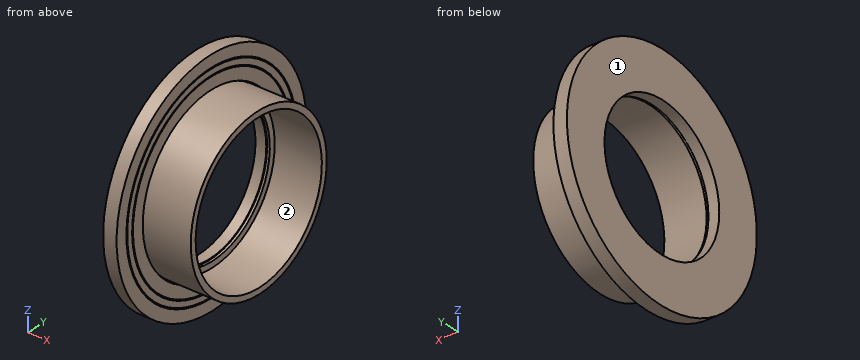
```python
from build123d import *

# Parameters (mm, degrees)
SKETCH1_R           = 17.08
SKETCH1_R_2         = 10.32
BOSS_EXTRUDE1_DEPTH = 2
SKETCH2_R           = 12.23
SKETCH2_R_2         = 11.35
BOSS_EXTRUDE2_DEPTH = 7
SKETCH3_R           = 10.47
SKETCH3_R_2         = 10.32
CUT_EXTRUDE1_DEPTH  = 0.4
SKETCH12_R          = 12.38
SKETCH12_R_2        = 12.23
CUT_EXTRUDE7_DEPTH  = 0.4
SKETCH13_R          = 14.29
SKETCH13_R_2        = 14.14
CUT_EXTRUDE8_DEPTH  = 0.4
SKETCH14_R          = 15.32
SKETCH14_R_2        = 15.17
CUT_EXTRUDE9_DEPTH  = 0.4


with BuildPart() as part:
    # Sketch1 → Boss-Extrude1 (new body)
    with BuildSketch(Plane(origin=(0, 0, 0), x_dir=(0, 0, -1), z_dir=(1, 0, 0))):
        Circle(SKETCH1_R)
        Circle(SKETCH1_R_2, mode=Mode.SUBTRACT)
    extrude(amount=BOSS_EXTRUDE1_DEPTH)

    # Sketch2 → Boss-Extrude2 (add)
    with BuildSketch(Plane(origin=(2, 0, 0), x_dir=(0, 0, -1), z_dir=(1, 0, 0))):
        Circle(SKETCH2_R)
        Circle(SKETCH2_R_2, mode=Mode.SUBTRACT)
    extrude(amount=BOSS_EXTRUDE2_DEPTH)

    # Sketch3 → Cut-Extrude1 (cut)
    with BuildSketch(Plane(origin=(2, 0, 0), x_dir=(0, 0, -1), z_dir=(1, 0, 0))):
        Circle(SKETCH3_R)
        Circle(SKETCH3_R_2, mode=Mode.SUBTRACT)
    extrude(amount=-CUT_EXTRUDE1_DEPTH, mode=Mode.SUBTRACT)

    # Sketch12 → Cut-Extrude7 (cut)
    with BuildSketch(Plane(origin=(2, 0, 0), x_dir=(0, 0, -1), z_dir=(1, 0, 0))):
        Circle(SKETCH12_R)
        Circle(SKETCH12_R_2, mode=Mode.SUBTRACT)
    extrude(amount=-CUT_EXTRUDE7_DEPTH, mode=Mode.SUBTRACT)

    # Sketch13 → Cut-Extrude8 (cut)
    with BuildSketch(Plane(origin=(2, 0, 0), x_dir=(0, 0, -1), z_dir=(1, 0, 0))):
        Circle(SKETCH13_R)
        Circle(SKETCH13_R_2, mode=Mode.SUBTRACT)
    extrude(amount=-CUT_EXTRUDE8_DEPTH, mode=Mode.SUBTRACT)

    # Sketch14 → Cut-Extrude9 (cut)
    with BuildSketch(Plane(origin=(2, 0, 0), x_dir=(0, 0, -1), z_dir=(1, 0, 0))):
        Circle(SKETCH14_R)
        Circle(SKETCH14_R_2, mode=Mode.SUBTRACT)
    extrude(amount=-CUT_EXTRUDE9_DEPTH, mode=Mode.SUBTRACT)


solid = part.part
```
Here's how the part is built. I have some questions about the finished solid (model axes, mm). Face numbers are marked on the shaded views. Give positions to 0.01 mm unless a question says otherwise; leave off trailing zeros. Write each loop counter-clockwise with the first axis right and the second up, starting at its lowest first coordinate (ties: lowest second). Pieces come first, ordered by that corner, then holes. Notation, with made-up numbers: M -10,6.5 L 28,6.5 A9 cw 28,11.5 Z; hole C -22.75,0 d6. An arc over 180 degrees is marked long. Put each result on its own line as item: value. Start each with the question number.
Item 1: I need wall thicknesses on L1, parallel to Y at x = 7.25, z = 0; L2, parallel to X at y = 13, z = -7; L3, parallel to Z at x = 4.5, y = -0.5. Which ranges of each line are inside material? Lowest first, please. Write a range as from..to.
Item 2: Thinking about a two-plate mould opening in Y: for the marked faces 1 and 2, which applies, +Y half, -Y half, draft (parallel to the pull), parting line (faces both ways), or undercut?
Item 3: If we section it at A-A, the plane x = 3.5: Write out the boundary of the cut face in (y, z).
Item 4: If we section it at B-B, the plane x = 1: Write out the boundary of the cut face in (y, z), then the cut area to 3 significant figures.
Item 5: Will these pins go through, and if not, where does the flat tip stop? pin 1 (1 mm diameter, centred on y = 9, z = -12.5, fed in from +X); pin 2 (14.5 mm diameter, centred on y = 0.5, z = -6, fed in from +X); pin 3 (4 mm diameter, centred on x = 5, z = -10, fed in from +Y); pin 4 (3 mm diameter, centred on x = 7.5, z = -3, fed in from +Y).
Values:
1. L1: -12.23..-11.35, 11.35..12.23
1. L2: 0..2
1. L3: -12.22..-11.34, 11.34..12.22
2. face 1: draft
2. face 2: undercut
3. outline: C 0,0 d24.46; hole C 0,0 d22.7
4. outline: C 0,0 d34.16; hole C 0,0 d20.64
4. area: 582 mm²
5. pin 1: x = 2
5. pin 2: x = 9
5. pin 3: y = 9.25
5. pin 4: y = 12.14
